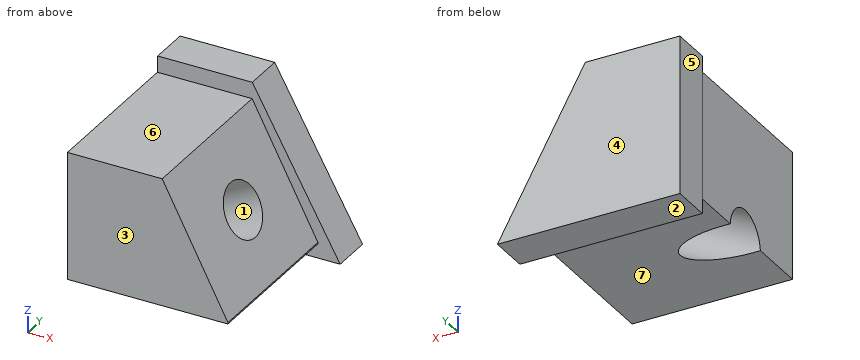
from build123d import *

# Parameters (mm, degrees)
F0_W      = 101.9186489284
F0_H      = 107.1304008365
F1_DEPTH  = 101.6
F3_DEPTH  = 101.9196489284
F5_DEPTH  = 101.9196489284
F6_R      = 17.1624207675
F7_DEPTH  = 90.5480102046
F10_DEPTH = 25.4


with BuildPart() as f1:
    # F0 (on Right) → F1 (new body)
    with BuildSketch(Plane.YZ):
        with Locations((-2.605875954, -0.1930259168)):
            Rectangle(F0_W, F0_H)
    extrude(amount=-F1_DEPTH)

    # F2 (on face) → F3 (cut, through all)
    with BuildSketch(Plane.XZ.offset(53.5652004182)):
        Polygon((13.0692059174, 68.6213597655), (-55.2626177669, 53.3721745014), (9.4016781077, -70.9377005696), align=None)
    extrude(amount=-F3_DEPTH, mode=Mode.SUBTRACT)

    # F4 (on face) → F5 (cut, through all)
    with BuildSketch(Plane.XZ.offset(53.5652004182)):
        Polygon((-121.2781071663, 53.3721745014), (-122.0502182841, 27.1203983575), (-16.0779859871, 27.1203983575), (-20.7106489688, 66.1120042205), align=None)
    extrude(amount=-F5_DEPTH, mode=Mode.SUBTRACT)

    # F6 (on face) → F7 (cut, through all)
    with BuildSketch(Plane(origin=(-21.6427491721, 0, -11.2582619458), x_dir=(0, 1, 0), z_dir=(0.8871491354, 0, 0.4614828399))):
        with Locations((0, -2.6491538156)):
            Circle(F6_R)
    extrude(amount=-F7_DEPTH, mode=Mode.SUBTRACT)

    # F9 (on face) → F10 (join)
    with BuildSketch(Plane(origin=(0, 48.3534485102, 0), x_dir=(-1, 0, 0), z_dir=(0, 1, 0))):
        Polygon((101.431466639, -54.2247891426), (101.431466639, 37.5402383506), (41.5187701583, 37.5402383506), (-14.0963997692, -62.819853425), (101.431466639, -62.819853425), align=None)
    extrude(amount=F10_DEPTH)


solid = f1.part
Verification items for the finished model (mm, model axes). Face numbers are marked on the shaded views. A direction names the side the tool comes from. Give positions to 0.01 mm unless a question says otherwise; leave off trailing zeros. Loops run counter-clockwise (first coordinate to the right, second up) from the corner with the lowest first, then second, coordinate; pieces in that order, holes last. Notation, with made-up numbers: (69, -12) - (83, -12) arc R16 ccw to (83, 5) - close; hole circle Ø10 at (-38, 77). An arc over 180 degrees is marked (long way). Write each question's results on one line, items separated by ' | '.
1) Material ranges on L1, parallel to Z at x = -67, y = 43; L2, parallel to Y at x = -24.5, z = 3; L3, parallel to Z at x = -60, y = 3, recorded low to high. Write a range as from..to.
Solution:
L1: -53.76..27.12 | L2: 48.35..73.75 | L3: -53.76..-53.25, -15.15..27.12
2) Sectioned sample at B-B on x = -4. Record the boundary of the cut face in (y, z).
Solution:
outline: (-53.57, -53.76) - (48.35, -53.76) - (48.35, -62.82) - (73.75, -62.82) - (73.75, -30.16) - (48.35, -30.16) - (48.35, -45.17) - (-53.57, -45.17) - close
3) Sectioned sample at C-C on y = 30. Record the boundary of the cut face in (x, z), plus the area to 3 significant figures.
Solution:
outline: (-101.6, -53.76) - (0, -53.76) - (0, -52.86) - (-41.61, 27.12) - (-101.6, 27.12) - close | area: 6,550 mm2
4) Sectioned sample at D-D on y = 3.5. Record the boundary of the cut face in (x, z).
Solution:
outline: (-101.6, -36.9) - (-28.17, 1.3) - (-41.61, 27.12) - (-101.6, 27.12) - close; (-61.2, -53.76) - (0, -53.76) - (0, -52.86) - (-12.67, -28.51) - close
5) Sectioned sample at A-A on y = -10. Record the boundary of the cut face in (x, z), plus the area to 3 significant figures.
Solution:
outline: (-101.6, -40.11) - (-26.86, -1.23) - (-41.61, 27.12) - (-101.6, 27.12) - close; (-67.38, -53.76) - (0, -53.76) - (0, -52.86) - (-13.98, -25.98) - close | area: 4,310 mm2
6) Mould release check, pull along Y, two halves, no side actions. Record for the marked faces 1, 2, 3 and 4: pulls with the +Y half, pulls with the -Y half, needs draft (parallel to the pull), parting line crosses it, or undercut.
Solution:
face 1: undercut | face 2: needs draft | face 3: pulls with the -Y half | face 4: pulls with the +Y half
7) Tool access check on the marked faces 5, 6 and 7. Record the directions out of +Z, -Z, +X, -X, +Y, -Y that give a thin tool (end or side, any length) a straight path to the whole face; none if there is none.
Solution:
face 5: +Z, -Z, -X, +Y | face 6: +Z, +X, -X, -Y | face 7: -Z, +X, -X, -Y
8) Depth check by flat-ended pin: P1, Ø12.5, axis at y = 65, z = -37, coming from the -X side; P2, Ø4, axis at x = -47.5, y = -18.5, coming from the -Z side; P3, Ø0.7, axis at y = 10.5, z = -53, coming from the +X side. Enter the tip coordinate at first touch or a pass-through.
Solution:
P1: x = -101.43 | P2: z = -53.76 | P3: x = 0
